from build123d import *

# Parameters (mm, degrees)
F0_W     = 717.99958
F0_H     = 738.954157
F1_DEPTH = 10.000005
F0_H_2   = 316.045765
F0_W_2   = 636.27
F0_H_3   = 227.04425
F2_DEPTH = 6.9088


with BuildPart() as f1:
    # F0 (on Top) → F1 (new body)
    with BuildSketch(Plane.XY):
        with Locations((358.99979, 369.477079)):
            Rectangle(F0_W, F0_H)
    extrude(amount=F1_DEPTH)

    # F0 (on Top) → F2 (join)
    with BuildSketch(Plane.XY):
        with Locations((358.99979, 896.97704)):
            Rectangle(F0_W, F0_H_2)
        with BuildLine():
            Line((12.28979, 769.497657), (24.98979, 769.497657))
            ThreePointArc((24.98979, 769.497657), (30.54604, 763.941407), (24.98979, 758.385157))
            Line((24.98979, 758.385157), (12.28979, 758.385157))
            ThreePointArc((12.28979, 758.385157), (6.73354, 763.941407), (12.28979, 769.497657))
        make_face(mode=Mode.SUBTRACT)
        with BuildLine():
            ThreePointArc((97.37979, 758.385157), (91.82354, 763.941407), (97.37979, 769.497657))
            Line((97.37979, 769.497657), (110.07979, 769.497657))
            ThreePointArc((110.07979, 769.497657), (115.63604, 763.941407), (110.07979, 758.385157))
            Line((110.07979, 758.385157), (97.37979, 758.385157))
        make_face(mode=Mode.SUBTRACT)
        with BuildLine():
            Line((195.16979, 758.385157), (182.46979, 758.385157))
            ThreePointArc((182.46979, 758.385157), (176.91354, 763.941407), (182.46979, 769.497657))
            Line((182.46979, 769.497657), (195.16979, 769.497657))
            ThreePointArc((195.16979, 769.497657), (200.72604, 763.941407), (195.16979, 758.385157))
        make_face(mode=Mode.SUBTRACT)
        with BuildLine():
            ThreePointArc((267.55979, 758.385157), (262.00354, 763.941407), (267.55979, 769.497657))
            Line((267.55979, 769.497657), (280.25979, 769.497657))
            ThreePointArc((280.25979, 769.497657), (285.81604, 763.941407), (280.25979, 758.385157))
            Line((280.25979, 758.385157), (267.55979, 758.385157))
        make_face(mode=Mode.SUBTRACT)
        with BuildLine():
            ThreePointArc((24.98979, 837.363282), (30.54604, 831.807032), (24.98979, 826.250782))
            Line((24.98979, 826.250782), (12.28979, 826.250782))
            ThreePointArc((12.28979, 826.250782), (6.73354, 831.807032), (12.28979, 837.363282))
            Line((12.28979, 837.363282), (24.98979, 837.363282))
        make_face(mode=Mode.SUBTRACT)
        with BuildLine():
            Line((12.28979, 905.228907), (24.98979, 905.228907))
            ThreePointArc((24.98979, 905.228907), (30.54604, 899.672657), (24.98979, 894.116407))
            Line((24.98979, 894.116407), (12.28979, 894.116407))
            ThreePointArc((12.28979, 894.116407), (6.73354, 899.672657), (12.28979, 905.228907))
        make_face(mode=Mode.SUBTRACT)
        with BuildLine():
            Line((12.28979, 973.094532), (24.98979, 973.094532))
            ThreePointArc((24.98979, 973.094532), (30.54604, 967.538282), (24.98979, 961.982032))
            Line((24.98979, 961.982032), (12.28979, 961.982032))
            ThreePointArc((12.28979, 961.982032), (6.73354, 967.538282), (12.28979, 973.094532))
        make_face(mode=Mode.SUBTRACT)
        with BuildLine():
            ThreePointArc((12.28979, 1029.847657), (6.73354, 1035.403907), (12.28979, 1040.960157))
            Line((12.28979, 1040.960157), (24.98979, 1040.960157))
            ThreePointArc((24.98979, 1040.960157), (30.54604, 1035.403907), (24.98979, 1029.847657))
            Line((24.98979, 1029.847657), (12.28979, 1029.847657))
        make_face(mode=Mode.SUBTRACT)
        with BuildLine():
            Line((97.37979, 1040.960157), (110.07979, 1040.960157))
            ThreePointArc((110.07979, 1040.960157), (115.63604, 1035.403907), (110.07979, 1029.847657))
            Line((110.07979, 1029.847657), (97.37979, 1029.847657))
            ThreePointArc((97.37979, 1029.847657), (91.82354, 1035.403907), (97.37979, 1040.960157))
        make_face(mode=Mode.SUBTRACT)
        with BuildLine():
            ThreePointArc((195.16979, 1040.960157), (200.72604, 1035.403907), (195.16979, 1029.847657))
            Line((195.16979, 1029.847657), (182.46979, 1029.847657))
            ThreePointArc((182.46979, 1029.847657), (176.91354, 1035.403907), (182.46979, 1040.960157))
            Line((182.46979, 1040.960157), (195.16979, 1040.960157))
        make_face(mode=Mode.SUBTRACT)
        with BuildLine():
            ThreePointArc((267.55979, 1029.847657), (262.00354, 1035.403907), (267.55979, 1040.960157))
            Line((267.55979, 1040.960157), (280.25979, 1040.960157))
            ThreePointArc((280.25979, 1040.960157), (285.81604, 1035.403907), (280.25979, 1029.847657))
            Line((280.25979, 1029.847657), (267.55979, 1029.847657))
        make_face(mode=Mode.SUBTRACT)
        with BuildLine():
            ThreePointArc((352.64979, 758.385157), (347.09354, 763.941407), (352.64979, 769.497657))
            Line((352.64979, 769.497657), (365.34979, 769.497657))
            ThreePointArc((365.34979, 769.497657), (370.90604, 763.941407), (365.34979, 758.385157))
            Line((365.34979, 758.385157), (352.64979, 758.385157))
        make_face(mode=Mode.SUBTRACT)
        with BuildLine():
            Line((437.73979, 769.497657), (450.43979, 769.497657))
            ThreePointArc((450.43979, 769.497657), (455.99604, 763.941407), (450.43979, 758.385157))
            Line((450.43979, 758.385157), (437.73979, 758.385157))
            ThreePointArc((437.73979, 758.385157), (432.18354, 763.941407), (437.73979, 769.497657))
        make_face(mode=Mode.SUBTRACT)
        with BuildLine():
            Line((535.52979, 758.385157), (522.82979, 758.385157))
            ThreePointArc((522.82979, 758.385157), (517.27354, 763.941407), (522.82979, 769.497657))
            Line((522.82979, 769.497657), (535.52979, 769.497657))
            ThreePointArc((535.52979, 769.497657), (541.08604, 763.941407), (535.52979, 758.385157))
        make_face(mode=Mode.SUBTRACT)
        with BuildLine():
            Line((620.61979, 758.385157), (607.91979, 758.385157))
            ThreePointArc((607.91979, 758.385157), (602.36354, 763.941407), (607.91979, 769.497657))
            Line((607.91979, 769.497657), (620.61979, 769.497657))
            ThreePointArc((620.61979, 769.497657), (626.17604, 763.941407), (620.61979, 758.385157))
        make_face(mode=Mode.SUBTRACT)
        with BuildLine():
            Line((705.70979, 758.385157), (693.00979, 758.385157))
            ThreePointArc((693.00979, 758.385157), (687.45354, 763.941407), (693.00979, 769.497657))
            Line((693.00979, 769.497657), (705.70979, 769.497657))
            ThreePointArc((705.70979, 769.497657), (711.26604, 763.941407), (705.70979, 758.385157))
        make_face(mode=Mode.SUBTRACT)
        with Locations((358.99979, 902.450782)):
            Rectangle(F0_W_2, F0_H_3, mode=Mode.SUBTRACT)
        with BuildLine():
            Line((365.34979, 1029.847657), (352.64979, 1029.847657))
            ThreePointArc((352.64979, 1029.847657), (347.09354, 1035.403907), (352.64979, 1040.960157))
            Line((352.64979, 1040.960157), (365.34979, 1040.960157))
            ThreePointArc((365.34979, 1040.960157), (370.90604, 1035.403907), (365.34979, 1029.847657))
        make_face(mode=Mode.SUBTRACT)
        with BuildLine():
            ThreePointArc((450.43979, 1040.960157), (455.99604, 1035.403907), (450.43979, 1029.847657))
            Line((450.43979, 1029.847657), (437.73979, 1029.847657))
            ThreePointArc((437.73979, 1029.847657), (432.18354, 1035.403907), (437.73979, 1040.960157))
            Line((437.73979, 1040.960157), (450.43979, 1040.960157))
        make_face(mode=Mode.SUBTRACT)
        with BuildLine():
            Line((535.52979, 1029.847657), (522.82979, 1029.847657))
            ThreePointArc((522.82979, 1029.847657), (517.27354, 1035.403907), (522.82979, 1040.960157))
            Line((522.82979, 1040.960157), (535.52979, 1040.960157))
            ThreePointArc((535.52979, 1040.960157), (541.08604, 1035.403907), (535.52979, 1029.847657))
        make_face(mode=Mode.SUBTRACT)
        with BuildLine():
            ThreePointArc((693.00979, 826.250782), (687.45354, 831.807032), (693.00979, 837.363282))
            Line((693.00979, 837.363282), (705.70979, 837.363282))
            ThreePointArc((705.70979, 837.363282), (711.26604, 831.807032), (705.70979, 826.250782))
            Line((705.70979, 826.250782), (693.00979, 826.250782))
        make_face(mode=Mode.SUBTRACT)
        with BuildLine():
            ThreePointArc((693.00979, 894.116407), (687.45354, 899.672657), (693.00979, 905.228907))
            Line((693.00979, 905.228907), (705.70979, 905.228907))
            ThreePointArc((705.70979, 905.228907), (711.26604, 899.672657), (705.70979, 894.116407))
            Line((705.70979, 894.116407), (693.00979, 894.116407))
        make_face(mode=Mode.SUBTRACT)
        with BuildLine():
            ThreePointArc((607.91979, 1029.847657), (602.36354, 1035.403907), (607.91979, 1040.960157))
            Line((607.91979, 1040.960157), (620.61979, 1040.960157))
            ThreePointArc((620.61979, 1040.960157), (626.17604, 1035.403907), (620.61979, 1029.847657))
            Line((620.61979, 1029.847657), (607.91979, 1029.847657))
        make_face(mode=Mode.SUBTRACT)
        with BuildLine():
            ThreePointArc((693.00979, 961.982032), (687.45354, 967.538282), (693.00979, 973.094532))
            Line((693.00979, 973.094532), (705.70979, 973.094532))
            ThreePointArc((705.70979, 973.094532), (711.26604, 967.538282), (705.70979, 961.982032))
            Line((705.70979, 961.982032), (693.00979, 961.982032))
        make_face(mode=Mode.SUBTRACT)
        with BuildLine():
            Line((705.70979, 1029.847657), (693.00979, 1029.847657))
            ThreePointArc((693.00979, 1029.847657), (687.45354, 1035.403907), (693.00979, 1040.960157))
            Line((693.00979, 1040.960157), (705.70979, 1040.960157))
            ThreePointArc((705.70979, 1040.960157), (711.26604, 1035.403907), (705.70979, 1029.847657))
        make_face(mode=Mode.SUBTRACT)
    extrude(amount=F2_DEPTH)


solid = f1.part
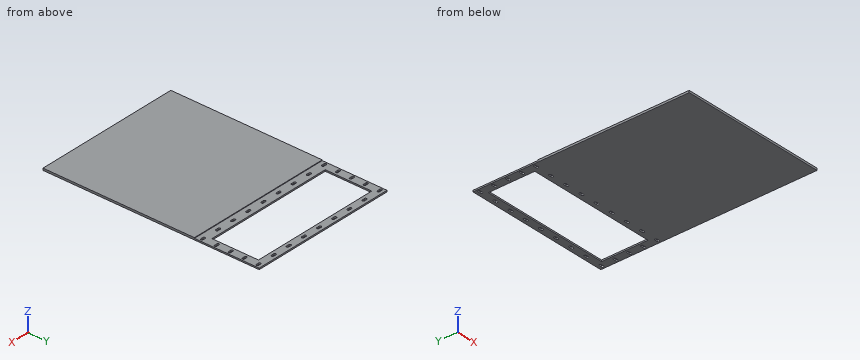
Could you check a few things on this model? Use its own coordinates, in mm. Round coordinates to 2 decimals unless told otherwise and drop trailing zeros. Write each loop counter-clockwise with the first axis right and the second up, starting at its lowest first coordinate (ties: lowest second). Pieces come first, ordered by that corner, then holes. Notation, with made-up numbers: (50, 82) - (95, 82) arc R23 ccw to (95, 99) - close; hole circle Ø11 at (72.25, 80). An arc over 180 degrees is marked (long way). Use a Markdown table: item, result.
Q1. I want a section at A-A (x = 159). List the corners of the cut face in (y, z) for me, plus the area to 3 significant figures.
Output values:
| item | result |
|---|---|
| outline | (0, 0) - (788.93, 0) - (788.93, 6.91) - (738.95, 6.91) - (738.95, 10) - (0, 10) - close; (1015.97, 0) - (1055, 0) - (1055, 6.91) - (1015.97, 6.91) - close |
| area | 8,000 mm2 |
Q2. Please list where these lines run through material, in increasing order: L1, parallel to Y at x = 354, z = 6.5; L2, parallel to X at y = 914, z = 3.5; L3, parallel to Y at x = 303, z = 4.25.
Output values:
| item | result |
|---|---|
| L1 | 0 to 758.39, 769.5 to 788.93, 1015.97 to 1029.85, 1040.96 to 1055 |
| L2 | 0 to 40.86, 677.13 to 718 |
| L3 | 0 to 788.93, 1015.97 to 1055 |
Q3. I want a section at B-B (z = 8.5). List the corners of the cut face in (x, y) for me.
Output values:
| item | result |
|---|---|
| outline | (0, 0) - (718, 0) - (718, 738.95) - (0, 738.95) - close |
